Here's how the part is built. I have some questions about the finished solid (model axes, mm). A direction names the side the tool comes from. Coordinates: 2 decimals unless noted, no trailing zeros. Loops run counter-clockwise (first coordinate to the right, second up) from the corner with the lowest first, then second, coordinate; pieces in that order, holes last. Notation, with made-up numbers: (14.5, -29) - (42.5, -29) arc R20 cw to (42.5, 0) - close; hole circle Ø11 at (-29, 23). An arc over 180 degrees is marked (long way). Use a Markdown table: item, result.
```python
from build123d import *

# Parameters (mm, degrees)
SKETCH1_W            = 30
SKETCH1_H            = 70
BOSS_EXTRUDE1_DEPTH  = 5
M5_CLEARANCE_HOLE1_D = 5.5
SKETCH4_W            = 5
SKETCH4_H            = 20
BOSS_EXTRUDE2_DEPTH  = 38.541999878
M5_CLEARANCE_HOLE2_D = 5.3
FILLET1_R            = 3
FILLET2_R            = 1
FILLET3_R            = 1
FILLET4_R            = 1
FILLET5_R            = 1
FILLET6_R            = 1


with BuildPart() as part:
    # Sketch1 → Boss-Extrude1 (new body)
    with BuildSketch(Plane.XY):
        Rectangle(SKETCH1_W, SKETCH1_H)
    extrude(amount=BOSS_EXTRUDE1_DEPTH)

    # M5 Clearance Hole1 (through all)
    with Locations(Plane.XY.offset(5)):
        with Locations((0, -23), (-7, 10), (7, 10)):
            Hole(M5_CLEARANCE_HOLE1_D / 2)

    # Sketch4 → Boss-Extrude2 (add)
    with BuildSketch(Plane.XY.offset(5)):
        with Locations((-12.5, 25)):
            Rectangle(SKETCH4_W, SKETCH4_H)
        with Locations((12.5, 25)):
            Rectangle(SKETCH4_W, SKETCH4_H)
    extrude(amount=BOSS_EXTRUDE2_DEPTH)

    # M5 Clearance Hole2 (through all)
    with Locations(Plane.ZY.offset(15)):
        with Locations((35.052, 25)):
            Hole(M5_CLEARANCE_HOLE2_D / 2)

    # Fillet1
    fillet1_edges = [part.edges().sort_by_distance(p)[0] for p in [
        (-10, 25, 5),
        (10, 25, 5),
    ]]
    fillet(fillet1_edges, radius=FILLET1_R)

    # Fillet2
    fillet2_edges = [part.edges().sort_by_distance(p)[0] for p in [
        (-15, 25, 43.541999878),
        (-10, 25, 43.541999878),
    ]]
    fillet(fillet2_edges, radius=FILLET2_R)

    # Fillet3
    # the kernel refuses this fillet: 1 mm, written as the material it takes off along each edge
    with BuildSketch(Plane(origin=(7, 15, 8), x_dir=(-0.7404019062872322, 0, -0.6721644271800112), z_dir=(-0.6721644271800112, 0, 0.7404019062872322))) as fillet3_piece_1_section:
        with BuildLine():
            CenterArc((3 + FILLET3_R, -FILLET3_R), FILLET3_R, 90, 90)
            Line((3 + FILLET3_R, 0), (3, 0))
            Line((3, 0), (3, -FILLET3_R))
        make_face()
    fillet3_piece_1 = revolve(axis=Axis((7, 15, 8), (0, -1, 0)), revolution_arc=137.765663079, mode=Mode.PRIVATE)
    fillet3_piece_1 = split(fillet3_piece_1, bisect_by=Plane(origin=(9.145909212, 15.257974559, 5), z_dir=(0, 0, 1)), keep=Keep.TOP, mode=Mode.PRIVATE)
    add(fillet3_piece_1, mode=Mode.SUBTRACT)
    with BuildSketch(Plane(origin=(-7, 15, 8), x_dir=(0.7404019062872333, 0, -0.6721644271800099), z_dir=(0.6721644271800099, 0, 0.7404019062872333))) as fillet3_piece_2_section:
        with BuildLine():
            CenterArc((3 + FILLET3_R, FILLET3_R), FILLET3_R, 180, 90)
            Line((3 + FILLET3_R, 0), (3, 0))
            Line((3, 0), (3, FILLET3_R))
        make_face()
    fillet3_piece_2 = revolve(axis=Axis((-7, 15, 8), (0, 1, 0)), revolution_arc=137.765663079, mode=Mode.PRIVATE)
    fillet3_piece_2 = split(fillet3_piece_2, bisect_by=Plane(origin=(-9.145909903, 15.257974038, 5), z_dir=(0, 0, 1)), keep=Keep.TOP, mode=Mode.PRIVATE)
    add(fillet3_piece_2, mode=Mode.SUBTRACT)
    with BuildSketch(Plane(origin=(-10, 15, 8), x_dir=(0, 1, 0), z_dir=(0, 0, 1))) as fillet3_piece_3:
        with BuildLine():
            CenterArc((FILLET3_R, FILLET3_R), FILLET3_R, 180, 90)
            Line((0, FILLET3_R), (0, 0))
            Line((0, 0), (FILLET3_R, 0))
        make_face()
    extrude(amount=34.541999878, mode=Mode.SUBTRACT)
    with BuildSketch(Plane(origin=(-11, 15, 42.541999878), x_dir=(1, 0, 0), z_dir=(0, 0, -1))) as fillet3_piece_4:
        with BuildLine():
            CenterArc((1 - FILLET3_R, -FILLET3_R), FILLET3_R, 0, 90)
            Line((1 - FILLET3_R, 0), (1, 0))
            Line((1, 0), (1, -FILLET3_R))
        make_face()
    revolve(axis=Axis((-11, 15, 42.541999878), (0, -1, 0)), revolution_arc=90, mode=Mode.SUBTRACT)
    with BuildSketch(Plane(origin=(-11, 15, 43.541999878), x_dir=(0, 0, -1), z_dir=(-1, 0, 0)), Plane(origin=(-14, 35, 43.541999878), x_dir=(0, 0, -1), z_dir=(1, 0, 0))) as fillet3_piece_5:
        with BuildLine():
            CenterArc((FILLET3_R, -FILLET3_R), FILLET3_R, 90, 90)
            Line((0, -FILLET3_R), (0, 0))
            Line((0, 0), (FILLET3_R, 0))
        make_face()
    extrude(amount=3, mode=Mode.SUBTRACT)
    with BuildSketch(Plane(origin=(-14, 15, 42.541999878), x_dir=(0, 0, 1), z_dir=(1, 0, 0))) as fillet3_piece_6:
        with BuildLine():
            CenterArc((1 - FILLET3_R, -FILLET3_R), FILLET3_R, 0, 90)
            Line((1, -FILLET3_R), (1, 0))
            Line((1, 0), (1 - FILLET3_R, 0))
        make_face()
    revolve(axis=Axis((-14, 15, 42.541999878), (0, -1, 0)), revolution_arc=90, mode=Mode.SUBTRACT)
    with BuildSketch(Plane(origin=(7, 35, 8), x_dir=(0, 0, -1), z_dir=(-1, 0, 0))) as fillet3_piece_7:
        with BuildLine():
            CenterArc((3 + FILLET3_R, FILLET3_R), FILLET3_R, 180, 90)
            Line((3, FILLET3_R), (3, 0))
            Line((3, 0), (3 + FILLET3_R, 0))
        make_face()
    revolve(axis=Axis((7, 35, 8), (0, -1, 0)), revolution_arc=90, mode=Mode.SUBTRACT)
    with BuildSketch(Plane(origin=(-7, 35, 5), x_dir=(0, 0, -1), z_dir=(1, 0, 0))) as fillet3_piece_8:
        with BuildLine():
            CenterArc((FILLET3_R, -FILLET3_R), FILLET3_R, 90, 90)
            Line((0, -FILLET3_R), (0, 0))
            Line((0, 0), (FILLET3_R, 0))
        make_face()
    extrude(amount=14, mode=Mode.SUBTRACT)
    with BuildSketch(Plane(origin=(-7, 35, 8), x_dir=(0, 0, -1), z_dir=(1, 0, 0))) as fillet3_piece_9:
        with BuildLine():
            CenterArc((3 + FILLET3_R, -FILLET3_R), FILLET3_R, 90, 90)
            Line((3, -FILLET3_R), (3, 0))
            Line((3, 0), (3 + FILLET3_R, 0))
        make_face()
    revolve(axis=Axis((-7, 35, 8), (0, 1, 0)), revolution_arc=90, mode=Mode.SUBTRACT)
    with BuildSketch(Plane(origin=(-10, 35, 8), x_dir=(0, -1, 0), z_dir=(0, 0, 1))) as fillet3_piece_10:
        with BuildLine():
            CenterArc((FILLET3_R, -FILLET3_R), FILLET3_R, 90, 90)
            Line((0, -FILLET3_R), (0, 0))
            Line((0, 0), (FILLET3_R, 0))
        make_face()
    extrude(amount=34.541999878, mode=Mode.SUBTRACT)
    with BuildSketch(Plane(origin=(-11, 35, 42.541999878), x_dir=(1, 0, 0), z_dir=(0, 0, -1))) as fillet3_piece_11:
        with BuildLine():
            CenterArc((1 - FILLET3_R, FILLET3_R), FILLET3_R, 270, 90)
            Line((1, FILLET3_R), (1, 0))
            Line((1, 0), (1 - FILLET3_R, 0))
        make_face()
    revolve(axis=Axis((-11, 35, 42.541999878), (0, -1, 0)), revolution_arc=90, mode=Mode.SUBTRACT)
    with BuildSketch(Plane(origin=(-14, 35, 42.541999878), x_dir=(0, 0, 1), z_dir=(1, 0, 0))) as fillet3_piece_12:
        with BuildLine():
            CenterArc((1 - FILLET3_R, FILLET3_R), FILLET3_R, 270, 90)
            Line((1, FILLET3_R), (1, 0))
            Line((1, 0), (1 - FILLET3_R, 0))
        make_face()
    revolve(axis=Axis((-14, 35, 42.541999878), (0, -1, 0)), revolution_arc=90, mode=Mode.SUBTRACT)
    with BuildSketch(Plane(origin=(10, 35, 8), x_dir=(1, 0, 0), z_dir=(0, 0, 1)), Plane(origin=(10, 15, 8), x_dir=(0, 1, 0), z_dir=(0, 0, 1))) as fillet3_piece_13:
        with BuildLine():
            CenterArc((FILLET3_R, -FILLET3_R), FILLET3_R, 90, 90)
            Line((0, -FILLET3_R), (0, 0))
            Line((0, 0), (FILLET3_R, 0))
        make_face()
    extrude(amount=38.041999878, mode=Mode.SUBTRACT)
    with BuildSketch(Plane(origin=(-15, 15, 5), x_dir=(1, 0, 0), z_dir=(0, 0, 1))) as fillet3_piece_14:
        with BuildLine():
            CenterArc((FILLET3_R, FILLET3_R), FILLET3_R, 180, 90)
            Line((0, FILLET3_R), (0, 0))
            Line((0, 0), (FILLET3_R, 0))
        make_face()
    extrude(amount=37.541999878, mode=Mode.SUBTRACT)
    with BuildSketch(Plane(origin=(-15, 35, 42.541999878), x_dir=(1, 0, 0), z_dir=(0, 0, -1))) as fillet3_piece_15:
        with BuildLine():
            CenterArc((FILLET3_R, FILLET3_R), FILLET3_R, 180, 90)
            Line((0, FILLET3_R), (0, 0))
            Line((0, 0), (FILLET3_R, 0))
        make_face()
    extrude(amount=45.041999878, mode=Mode.SUBTRACT)

    # Fillet4
    fillet4_edges = [part.edges().sort_by_distance(p)[0] for p in [
        (15, 15, 24.270999939),
        (15, 35, 21.770999939),
    ]]
    fillet(fillet4_edges, radius=FILLET4_R)

    # Fillet5
    fillet5_edges = [part.edges().sort_by_distance(p)[0] for p in [
        (-15, -9.5, 5),
        (15, -9.5, 5),
    ]]
    fillet(fillet5_edges, radius=FILLET5_R)

    # Fillet6
    fillet6_edges = [part.edges().sort_by_distance(p)[0] for p in [
        (0, -35, 5),
        (15, -35, 2),
        (-15, -35, 2),
        (14.707106781, -35, 4.707106781),
        (-14.707106781, -35, 4.707106781),
    ]]
    fillet(fillet6_edges, radius=FILLET6_R)


solid = part.part
```
Q1. I want a section at B-B, the plane y = 25. Write out the boundary of the cut face in (x, z), then the cut area to 3 significant figures.
Check values:
| item | result |
|---|---|
| outline | (-15, 0) - (15, 0) - (15, 32.4) - (10, 32.4) - (10, 8) arc R3 cw to (7, 5) - (-7, 5) arc R3 cw to (-10, 8) - (-10, 32.4) - (-15, 32.4) - close; (-15, 37.7) - (-10, 37.7) - (-10, 42.54) arc R1 ccw to (-11, 43.54) - (-14, 43.54) arc R1 ccw to (-15, 42.54) - close; (10, 37.7) - (15, 37.7) - (15, 43.54) - (10, 43.54) - close |
| area | 486 mm^2 |
Q2. I want a section at A-A, the plane z = 29.5. Write out the boundary of the cut face in (x, y).
Check values:
| item | result |
|---|---|
| outline | (-15, 16) arc R1 ccw to (-14, 15) - (-11, 15) arc R1 ccw to (-10, 16) - (-10, 34) arc R1 ccw to (-11, 35) - (-14, 35) arc R1 ccw to (-15, 34) - close; (10, 16) arc R1 ccw to (11, 15) - (14, 15) arc R1 ccw to (15, 16) - (15, 34) arc R1 ccw to (14, 35) - (11, 35) arc R1 ccw to (10, 34) - close |
Q3. Which directions (+Z, -Z, +X, -X, +Y, -Y) give clear straight access to the entire face, cutting with the end or side of a thin tool? Please do faces 5 (the face through (10, 25, 26)), 6 (the face through (13, 15, 24)), 7 (the face through (0, -7, 5)).
Check values:
| item | result |
|---|---|
| face 5 | +Z, +Y, -Y |
| face 6 | +Z, +X, -X, -Y |
| face 7 | +Z, -Y |
Q4. I want a section at D-D, the plane y = -23. Write out the boundary of the cut face in (x, z), then the cut area to 3 significant figures.
Check values:
| item | result |
|---|---|
| outline | (-15, 0) - (-2.75, 0) - (-2.75, 5) - (-14, 5) arc R1 ccw to (-15, 4) - close; (2.75, 0) - (15, 0) - (15, 4) arc R1 ccw to (14, 5) - (2.75, 5) - close |
| area | 122 mm^2 |
Q5. If we mould it in two halves opening along Y, with no side actions, what happens to faces 1 (the face through (-12.465, 23.388, 37.155)), 2 (the face through (-12, 15, 24)), 3 (the face through (12.535, 23.388, 37.155)), 4 (the face through (-10, 25, 25))? For each: pulls with the +Y half, pulls with the -Y half, needs draft (parallel to the pull), parting line crosses it, or undercut.
Check values:
| item | result |
|---|---|
| face 1 | undercut |
| face 2 | pulls with the -Y half |
| face 3 | undercut |
| face 4 | needs draft |
Q6. I want a section at C-C, the plane x = -5.25. Write out the boundary of the cut face in (y, z), then the cut area to 3 significant figures.
Check values:
| item | result |
|---|---|
| outline | (-35, 0) - (7.88, 0) - (7.88, 5) - (-34, 5) arc R1 ccw to (-35, 4) - close; (12.12, 0) - (35, 0) - (35, 4) arc R1 ccw to (34, 5) - (12.12, 5) - close |
| area | 328 mm^2 |
Q7. Will these pins go through, and if not, where does the flat tip stop? P1, Ø3, axis at y = 25, z = 35.052, coming from the +X side; P2, Ø2, axis at x = -11.5, z = 14.5, coming from the -Y side; P3, Ø2, axis at x = -3, y = 17, coming from the -Z side; P4, Ø6.5, axis at x = -7, y = 10, coming from the +Z side.
Check values:
| item | result |
|---|---|
| P1 | through |
| P2 | y = 15 |
| P3 | z = 0 |
| P4 | z = 5 |
Q8. Please list where these lines run through material, in increasing order: L1, parallel to Y at x = -7, z = 3.45; L2, parallel to X at y = 22.5, z = 8; L3, parallel to Y at x = 0, z = 2.75. Write a range as from..to.
Check values:
| item | result |
|---|---|
| L1 | -35..7.25, 12.75..35 |
| L2 | -15..-10, 10..15 |
| L3 | -35..-25.75, -20.25..35 |
